```python
from build123d import *

# Parameters (mm, degrees)
BOSS_EXTRUDE1_DEPTH = 27.5
FILLET1_R           = 0.2


with BuildPart() as part:
    # Sketch1 → Boss-Extrude1 (new body)
    with BuildSketch(Plane(origin=(0, 0, 0), x_dir=(0, 0, -1), z_dir=(1, 0, 0))):
        with BuildLine():
            Line((-4.3133513652379465, 4.313351365237932), (-3.6000000000000107, 3.5999999999999988))
            Line((-3.6000000000000103, 3.5999999999999996), (-1.9621416870348378, 3.5999999999999996))
            ThreePointArc((-1.962141687034841, 3.6000000000000094), (-1.978e-14, 4.1), (1.962141687034806, 3.600000000000028))
            Line((1.9621416870347996, 3.5999999999999996), (4.924428900898164, 3.5999999999999996))
            ThreePointArc((4.9244289008981275, 3.5999999999998975), (4.632641104588721, 3.96845516493194), (4.3133513652379465, 4.313351365237932))
            ThreePointArc((4.3133513652379465, 4.313351365237932), (2.3343689374270524, 5.6356651483188465), (3.7e-16, 6.1))
            ThreePointArc((3.7e-16, 6.1), (-2.334368937427052, 5.6356651483188465), (-4.3133513652379465, 4.313351365237932))
        make_face()
        with BuildLine():
            Line((8, 6.1), (0, 6.1))
            ThreePointArc((3.7e-16, 6.1), (2.3343689374270524, 5.6356651483188465), (4.3133513652379465, 4.313351365237932))
            Line((4.3133513652379465, 4.313351365237932), (8, 4.313351365237933))
            Line((8, 4.313351365237933), (8, 6.1))
        make_face()
        with BuildLine():
            ThreePointArc((4.3133513652379465, 4.313351365237932), (4.632641104588721, 3.96845516493194), (4.9244289008981275, 3.5999999999998975))
            Line((4.924428900898164, 3.5999999999999996), (8, 3.5999999999999996))
            Line((8, 3.5999999999999996), (8, 4.313351365237933))
            Line((8, 4.313351365237933), (4.3133513652379465, 4.313351365237932))
        make_face()
        with BuildLine():
            Line((8, 3.5999999999999996), (4.924428900898164, 3.5999999999999996))
            ThreePointArc((4.9244289008981275, 3.5999999999998975), (5.7986643417031205, 1.8935395037497136), (6.1, 0))
            ThreePointArc((6.1, -1.49e-15), (5.7986643417031205, -1.8935395037497147), (4.924428900898127, -3.599999999999898))
            Line((4.924428900898162, -3.6), (8, -3.5999999999999996))
            Line((8, -3.5999999999999996), (8, 3.5999999999999996))
        make_face()
        with BuildLine():
            ThreePointArc((4.3133513652379465, -4.313351365237933), (2.334368937427049, -5.635665148318848), (-6.54e-15, -6.1))
            Line((-6.22e-15, -6.1), (8, -6.1))
            Line((8, -6.1), (8, -4.313351365237933))
            Line((8, -4.313351365237933), (4.3133513652379465, -4.313351365237932))
        make_face()
        with BuildLine():
            Line((8, -3.5999999999999996), (4.924428900898162, -3.6))
            ThreePointArc((4.924428900898127, -3.599999999999898), (4.6326411045887195, -3.968455164931942), (4.3133513652379465, -4.313351365237933))
            Line((4.3133513652379465, -4.313351365237932), (8, -4.313351365237933))
            Line((8, -4.313351365237933), (8, -3.5999999999999996))
        make_face()
        with BuildLine():
            Line((-1.9621416870348352, -3.6000000000000005), (-3.6000000000000156, -3.600000000000001))
            Line((-3.600000000000014, -3.6000000000000023), (-4.3133513652379465, -4.313351365237932))
            ThreePointArc((-4.313351365237948, -4.313351365237931), (-2.334368937427056, -5.635665148318846), (-6.54e-15, -6.1))
            ThreePointArc((-6.54e-15, -6.1), (2.334368937427049, -5.635665148318848), (4.3133513652379465, -4.313351365237933))
            ThreePointArc((4.3133513652379465, -4.313351365237933), (4.6326411045887195, -3.968455164931942), (4.924428900898127, -3.599999999999898))
            Line((4.924428900898162, -3.6), (1.9621416870348023, -3.6000000000000005))
            ThreePointArc((1.9621416870348085, -3.6000000000000267), (-1.532e-14, -4.1), (-1.9621416870348387, -3.6000000000000103))
        make_face()
    extrude(amount=BOSS_EXTRUDE1_DEPTH)

    # Fillet1
    fillet1_edges = [part.edges().sort_by_distance(p)[0] for p in [
        (0, -6.1, -3.9999999999999973),
        (0, -5.635665148318846, 2.334368937427055),
        (0, -3.9566756826189673, 3.95667568261898),
        (27.5, 6.1, -4),
        (0, -3.6000000000000005, 2.7810708435174254),
        (0, -4.1000000000000005, 1.654e-14),
        (0, -3.6, -3.443285293966482),
        (0, -6.1e-16, -6.100000000000001),
        (0, 3.6000000000000103, -3.4432852939664738),
        (0, 4.1, 1.982e-14),
        (0, 3.5999999999999996, 2.781070843517424),
        (0, 3.9566756826189655, 3.956675682618979),
        (0, 5.635665148318875, 2.334368937427066),
        (27.5, 5.6356651483188465, 2.334368937427051),
        (0, 6.1, -4),
        (0, 0, -8),
        (27.5, 3.9566756826189655, 3.956675682618979),
        (13.75, -6.1, -8),
        (13.75, -4.313351365237931, 4.313351365237947),
        (13.75, -3.6000000000000014, 3.6000000000000147),
        (13.75, -3.600000000000006, 1.9621416870348367),
        (13.75, -3.600000000000014, -1.9621416870348056),
        (13.75, -3.599999999999949, -4.924428900898144),
        (13.75, 3.599999999999948, -4.924428900898145),
        (13.75, 3.600000000000014, -1.9621416870348032),
        (13.75, 3.600000000000005, 1.9621416870348396),
        (13.75, 3.599999999999999, 3.6000000000000103),
        (13.75, 4.313351365237933, 4.313351365237946),
        (13.75, 6.1, -8),
        (27.5, 3.5999999999999996, 2.781070843517424),
        (27.5, 4.1, 1.982e-14),
        (27.5, 0, -8),
        (27.5, 3.6000000000000103, -3.4432852939664738),
        (27.5, -6.1e-16, -6.100000000000001),
        (27.5, -3.6, -3.443285293966482),
        (27.5, -4.1000000000000005, 1.654e-14),
        (27.5, -3.6000000000000005, 2.7810708435174254),
        (27.5, -3.9566756826189673, 3.95667568261898),
        (27.5, -5.635665148318815, 2.3343689374270387),
        (27.5, -6.1, -3.9999999999999973),
    ]]
    fillet(fillet1_edges, radius=FILLET1_R)


solid = part.part
```
Design review of the part built by this model. Coordinates are the model's own, in mm. A direction names the side the tool comes from. Coordinates: 2 decimals unless noted, no trailing zeros. Order: outer loops, then holes, each group sorted by start corner. A loop starts at its lowest first (then second) coordinate and runs counter-clockwise, first axis right, second up. Notation, with made-up numbers: M -35.5,-7 L -11.5,-7 A6 ccw -11.5,2 Z; hole C -14.5,-20.75 d5. An arc over 180 degrees is marked long. Answer as a JSON object with one key per item and string values. Group by question number.
1) For pin 1 (0.8 mm diameter, centred on x = 20, z = 3, fed in from +Y); pin 2 (1 mm diameter, centred on x = 8, z = 1, fed in from +Y); pin 3 (6 mm diameter, centred on x = 13, y = -0.5, fed in from +Z), all flat-tipped, find the tip position at first contact; note any pin that passes through.
2) Wall thickness on L1, parallel to Y at x = 23.25, z = -2.75; L2, parallel to Y at x = 8.25, z = 3; L3, parallel to Z at x = 16.75, y = 0: over which ranges is each line inside the solid? List them lowest first.
3) Mouldability with a two-part tool opening along Y and no side actions: class faces 1 (the flat face through (14, 6.1, -4)), 2 (the flat face through (14, -3.6, 3)), 3 (the cylindrical face through (13.6, 0.1, -6.1)), 4 (the flat face through (14, -6.1, -4)) as pulls with the +Y half, pulls with the -Y half, needs draft (parallel to the pull), parting line crosses it, or undercut.
4) Add section B-B, the plane x = 23.75. Write out the cut boundary in (y, z).
5) Add section A-A, the plane z = -2.5. Write out the cut boundary in (x, y).
6) Tool access review of faces 5 (the flat face through (14, 3.6, -3)), 6 (the flat face through (0, 3, -6)), 7 (the cylindrical face through (13.6, 4.1, 0)): name each direction out of +Z, -Z, +X, -X, +Y, -Y from which nothing blocks a thin tool from reaching the whole face with its end or side.
Computed values:
{
 "1": {"pin 1": "stops at y = 5.52", "pin 2": "stops at y = 6.08", "pin 3": "stops at z = -5"},
 "2": {"L1": "y = -6.1 to -3.6, 3.6 to 6.1", "L2": "y = -5.31 to -3.6, 3.6 to 5.31", "L3": "z = -8 to -6.1"},
 "3": {"face 1": "pulls with the +Y half", "face 2": "undercut", "face 3": "undercut", "face 4": "pulls with the -Y half"},
 "4": {"outline": "M -6.1,-7.8 A0.2 ccw -5.9,-8 L 5.9,-8 A0.2 ccw 6.1,-7.8 L 6.1,0 A6.1 ccw 4.46,4.16 A0.2 ccw 4.17,4.17 L 3.66,3.66 A0.2 ccw 3.6,3.52 L 3.6,2.01 A0.2 ccw 3.62,1.92 A4.1 cw 3.62,-1.92 A0.2 ccw 3.6,-2.01 L 3.6,-4.82 A0.2 cw 3.52,-4.99 A6.1 cw -3.52,-4.99 A0.2 cw -3.6,-4.82 L -3.6,-2.01 A0.2 ccw -3.62,-1.92 A4.1 cw -3.62,1.92 A0.2 ccw -3.6,2.01 L -3.6,3.52 A0.2 ccw -3.66,3.66 L -4.17,4.17 A0.2 ccw -4.46,4.16 A6.1 ccw -6.1,0 Z"},
 "5": {"outline": "M 0,-5.9 A0.2 ccw 0.2,-6.1 L 27.3,-6.1 A0.2 ccw 27.5,-5.9 L 27.5,-3.8 A0.2 ccw 27.3,-3.6 L 0.2,-3.6 A0.2 ccw 0,-3.8 Z; M 0,3.8 A0.2 ccw 0.2,3.6 L 27.3,3.6 A0.2 ccw 27.5,3.8 L 27.5,5.9 A0.2 ccw 27.3,6.1 L 0.2,6.1 A0.2 ccw 0,5.9 Z"},
 "6": {"face 5": "+Z, +X, -X", "face 6": "+Z, -Z, -X, +Y, -Y", "face 7": "+X, -X"}
}
